from build123d import *

# Parameters (mm, degrees)
F1_DEPTH  = 40
F2_R      = 3.25
F3_DEPTH  = 25
F4_R      = 3.25
F4_R_2    = 2
F5_DEPTH  = 25
F6_SIZE   = 5
F7_SIZE   = 5
F8_DEPTH  = 25
F9_W      = 50.789644
F9_H      = 57.590966
F10_DEPTH = 51.1
F11_SIZE  = 5
F12_SIZE  = 5
F13_R     = 4
F14_R     = 5


with BuildPart() as f1:
    # F0 (on Front) → F1 (new body)
    with BuildSketch(Plane.XZ):
        Polygon((0, 50), (0, 0), (50, 0), (50, 5), (5, 5), (5, 50), align=None)
    extrude(amount=F1_DEPTH)

    # F2 (on face) → F3 (cut)
    with BuildSketch(Plane(origin=(0, 0, 0), x_dir=(1, 0, 0), z_dir=(0, 0, -1))):
        with Locations((25, 20)):
            Circle(F2_R)
        with BuildLine():
            ThreePointArc((37.049758, 30.526316), (41, 20), (37.049758, 9.473684))
            ThreePointArc((37.049758, 9.473684), (37.335405, 5.240671), (41.568419, 5.526317))
            ThreePointArc((41.568419, 5.526317), (47, 20.000001), (41.568418, 34.473684))
            ThreePointArc((41.568418, 34.473684), (37.335404, 34.75933), (37.049758, 30.526316))
        make_face()
        with Locations((12.5, 20)):
            Circle(F2_R)
        with Locations((35, 20)):
            Circle(F2_R)
        with BuildLine():
            Line((26.554622, -9.521332), (37.049758, 0))
            ThreePointArc((37.049758, 0), (21.024879, 7.89477), (5, 0))
            Line((5, 0), (26.554622, -9.521332))
        make_face()
        with BuildLine():
            Line((21.024879, 52.316344), (5, 40))
            ThreePointArc((5, 40), (21.024879, 32.105231), (37.049758, 40))
            Line((37.049758, 40), (21.024879, 52.316344))
        make_face()
    extrude(amount=-F3_DEPTH, mode=Mode.SUBTRACT)

    # F4 (on face) → F5 (cut)
    with BuildSketch(Plane(origin=(0, 0, 0), x_dir=(0, -1, 0), z_dir=(-1, 0, 0))):
        with Locations((20, 12.5)):
            Circle(F4_R)
        with Locations((20, 25)):
            Circle(F4_R)
        with Locations((20, 35)):
            Circle(F4_R)
        with BuildLine():
            ThreePointArc((9.473684, 37.049758), (20, 41), (30.526316, 37.049758))
            ThreePointArc((30.526316, 37.049758), (34.75933, 37.335404), (34.473684, 41.568418))
            ThreePointArc((34.473684, 41.568418), (20, 47), (5.526316, 41.568418))
            ThreePointArc((5.526316, 41.568418), (5.24067, 37.335404), (9.473684, 37.049758))
        make_face()
        with Locations((32.5, 12.5)):
            Circle(F4_R_2)
        with Locations((32.5, 25)):
            Circle(F4_R_2)
        with Locations((7.5, 25)):
            Circle(F4_R_2)
        with Locations((7.5, 12.5)):
            Circle(F4_R_2)
    extrude(amount=-F5_DEPTH, mode=Mode.SUBTRACT)

    # F6
    f6_edges = [f1.edges().sort_by_distance(p)[0] for p in [
        (50, -40, 2.5),
    ]]
    chamfer(f6_edges, length=F6_SIZE)

    # F7
    f7_edges = [f1.edges().sort_by_distance(p)[0] for p in [
        (50, 0, 2.5),
    ]]
    chamfer(f7_edges, length=F7_SIZE)

    # F2 (on face) → F8 (cut)
    with BuildSketch(Plane(origin=(0, 0, 0), x_dir=(1, 0, 0), z_dir=(0, 0, -1))):
        with Locations((25, 20)):
            Circle(F2_R)
        with BuildLine():
            ThreePointArc((37.049758, 30.526316), (41, 20), (37.049758, 9.473684))
            ThreePointArc((37.049758, 9.473684), (37.335405, 5.240671), (41.568419, 5.526317))
            ThreePointArc((41.568419, 5.526317), (47, 20.000001), (41.568418, 34.473684))
            ThreePointArc((41.568418, 34.473684), (37.335404, 34.75933), (37.049758, 30.526316))
        make_face()
        with Locations((12.5, 20)):
            Circle(F2_R)
        with Locations((35, 20)):
            Circle(F2_R)
        with BuildLine():
            Line((26.554622, -9.521332), (37.049758, 0))
            ThreePointArc((37.049758, 0), (21.024879, 7.89477), (5, 0))
            Line((5, 0), (26.554622, -9.521332))
        make_face()
        with BuildLine():
            Line((21.024879, 52.316344), (5, 40))
            ThreePointArc((5, 40), (21.024879, 32.105231), (37.049758, 40))
            Line((37.049758, 40), (21.024879, 52.316344))
        make_face()
    extrude(amount=F8_DEPTH, mode=Mode.SUBTRACT)

    # F9 (on face) → F10 (cut)
    with BuildSketch(Plane.XZ.offset(40)):
        with Locations((28.394822, 31.795483)):
            Rectangle(F9_W, F9_H)
    extrude(amount=-F10_DEPTH, mode=Mode.SUBTRACT)

    # F11
    f11_edges = [f1.edges().sort_by_distance(p)[0] for p in [
        (1.5, 0, 50),
    ]]
    chamfer(f11_edges, length=F11_SIZE)

    # F12
    f12_edges = [f1.edges().sort_by_distance(p)[0] for p in [
        (1.5, -40, 50),
    ]]
    chamfer(f12_edges, length=F12_SIZE)

    # F13
    f13_edges = [f1.edges().sort_by_distance(p)[0] for p in [
        (3, -20, 3),
    ]]
    fillet(f13_edges, radius=F13_R)

    # F14
    f14_edges = [f1.edges().sort_by_distance(p)[0] for p in [
        (0, -20, 0),
    ]]
    fillet(f14_edges, radius=F14_R)


solid = f1.part
Design review of the part built by this model. Coordinates are the model's own, in mm. A direction names the side the tool comes from. Round coordinates to 2 decimals unless told otherwise and drop trailing zeros. Write each loop counter-clockwise with the first axis right and the second up, starting at its lowest first coordinate (ties: lowest second). Pieces come first, ordered by that corner, then holes. Notation, with made-up numbers: M 5,-20.5 L 54,-20.5 A23 cw 54,0.5 Z; hole C 44.25,10 d6. An arc over 180 degrees is marked long. One line per item, written item: value. Start each with the question number.
1. To check wall thickness, follow probe 1 along Y at (x, z) = (1, 12); probe 2 along Z at (x, y) = (1, -32); probe 3 along X at (y, z) = (-9, 28.5). State the ranges of each line that lie inside material, in increasing order. Write a range as from..to.
2. Take a section at C-C on x = 12.5. State the section outline as (y, z) points.
3. Take a section at B-B on z = 35. State the section outline as (x, y) points, then the cut area to 4 significant figures.
4. Take a section at A-A on z = 12.5. State the section outline as (x, y) points, then the cut area to 3 significant figures.
5. Clearance check with flat-ended pins moving along their axes: P1, Ø1, axis at y = -32.5, z = 8.5, coming from the +X side; P2, Ø1, axis at x = 30, y = -26.5, coming from the +Z side. State where each tip first meets the part, or that it passes through.
6. For faces 1 (the face through (27, -24, 0)), 2 (the face through (28, -16, 3)), list the 3-axis set-ups (+Z, -Z, +X, -X, +Y, -Y) from which the entire face can be reached by the end or side of a thin tool; tool diameter is ignored.
7. Draft analysis for pull direction Z (two halves, no side actions). For faces 3 (the face through (0, -15, 28)), 4 (the face through (2, -3, 48)), 5 (the face through (1.479, -34.408, 13.101)), 6 (the face through (1, -20, 41)), state which applies: pulls with the +Z half, pulls with the -Z half, needs draft (parallel to the pull), parting line crosses it, or undercut.
8. Take a section at D-D on x = 21. State the section outline as (y, z) points, then the cut area to 3 significant figures.
Computed:
1. probe 1: y = -40..-34.44, -30.56..-23.21, -16.79..-9.44, -5.56..0
1. probe 2: z = 2..10.56, 14.44..23.06, 26.94..36.35, 43.44..50
1. probe 3: x = 0..3
2. outline: M -33.99,0 L -23.25,0 L -23.25,3 L -33.99,3 Z; M -16.75,0 L -6.01,0 L -6.01,3 L -16.75,3 Z
3. outline: M 0,-40 L 3,-40 L 3,-23.25 L 0,-23.25 Z; M 0,-16.75 L 3,-16.75 L 3,0 L 0,0 Z
3. area: 100.5 mm²
4. outline: M 0,-40 L 3,-40 L 3,-34.5 L 0,-34.5 Z; M 0,-30.5 L 3,-30.5 L 3,-23.25 L 0,-23.25 Z; M 0,-16.75 L 3,-16.75 L 3,-9.5 L 0,-9.5 Z; M 0,-5.5 L 3,-5.5 L 3,0 L 0,0 Z
4. area: 76.5 mm²
5. P1: stops at x = 3
5. P2: stops at z = 3
6. face 1: -Z, +X, -X, +Y, -Y
6. face 2: +Z, +X, +Y, -Y
7. face 3: needs draft
7. face 4: pulls with the +Z half
7. face 5: undercut
7. face 6: undercut
8. outline: M -32.11,0 L -7.89,0 L -7.89,3 L -32.11,3 Z
8. area: 72.6 mm²
